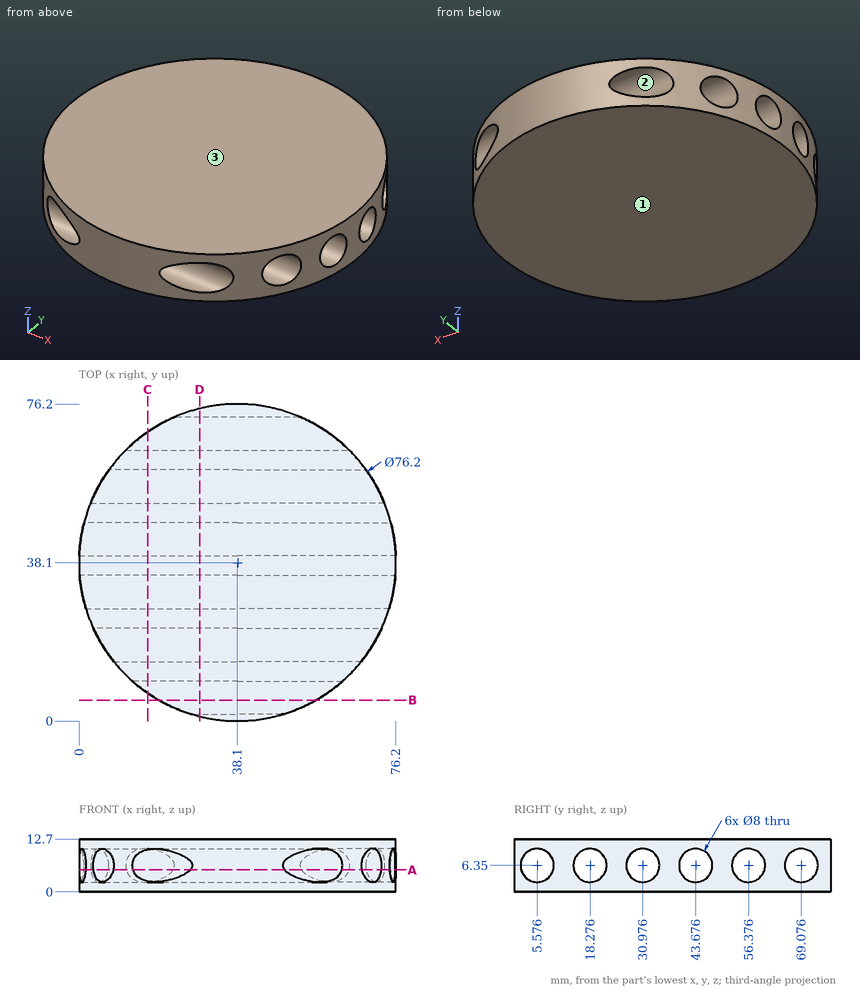
The drawing under review shows one solid part. Ordinate dimensions are in mm from its lowest x, y, z. Round coordinates to 2 decimals unless told otherwise and drop trailing zeros. Write each loop counter-clockwise with the first axis right and the second up, starting at its lowest first coordinate (ties: lowest second). Pieces come first, ordered by that corner, then holes. Notation, with made-up numbers: (15, 35.25) - (36, 35.25) arc R11 ccw to (36, 52.25) - close; hole circle Ø6 at (-37.5, 34). An arc over 180 degrees is marked (long way). One line per question, with ' | ' between items.
Item 1: The part is to be moulded in two halves that separate along Z. For the marked faces 1, 2 and 3, say which applies: pulls with the +Z half, pulls with the -Z half, needs draft (parallel to the pull), parting line crosses it, or undercut.
Resolved:
face 1: pulls with the -Z half | face 2: undercut | face 3: pulls with the +Z half
Item 2: Add section B-B, the plane y = 5. Give the boundary of the cut face in (x, z), then the cut area to 4 significant figures.
Resolved:
outline: (19.23, 0) - (56.97, 0) - (56.97, 2.39) - (19.23, 2.39) - close; (19.23, 10.31) - (56.97, 10.31) - (56.97, 12.7) - (19.23, 12.7) - close | area: 180.5 mm2
Item 3: To check wall thickness, follow probe 1 along Y at (x, z) = (72, 5); probe 2 along Y at (x, z) = (10.5, 5.25) (1 decimal); probe 3 along Y at (x, z) = (57, 7.75). State the ranges of each line that lie inside material, in increasing order.
Resolved:
probe 1: y = 22.04 to 27.21, 34.74 to 39.91, 47.44 to 52.61 | probe 2: y = 11.8 to 14.4, 22.1 to 27.1, 34.8 to 39.8, 47.5 to 52.5, 60.2 to 64.4 | probe 3: y = 9.32 to 14.53, 22.02 to 27.23, 34.72 to 39.93, 47.42 to 52.63, 60.12 to 65.33
Item 4: Add section A-A, the plane z = 5.25. Give the boundary of the cut face in (x, y).
Resolved:
outline: (0.04, 39.83) arc R38.1 ccw to (0.14, 34.82) - (76.06, 34.82) arc R38.1 ccw to (76.16, 39.83) - close; (1.18, 47.52) - (75.02, 47.52) arc R38.1 ccw to (73.36, 52.53) - (2.84, 52.53) arc R38.1 ccw to start; (1.61, 27.13) arc R38.1 ccw to (3.51, 22.12) - (72.69, 22.12) arc R38.1 ccw to (74.59, 27.13) - close; (7.08, 60.22) - (69.12, 60.22) arc R38.1 ccw to (64.85, 65.23) - (11.35, 65.23) arc R38.1 ccw to start; (8.24, 14.43) arc R38.1 ccw to (13.02, 9.42) - (63.18, 9.42) arc R38.1 ccw to (67.96, 14.43) - close; (22.64, 72.92) - (53.56, 72.92) arc R38.1 ccw to start; (26.75, 1.73) arc R38.1 ccw to (49.45, 1.73) - close
Item 5: Add section C-C, the plane x = 16.5. Give the boundary of the cut face in (y, z), then the cut area to 3 significant figures.
Resolved:
outline: (6.71, 0) - (69.49, 0) - (69.49, 2.37) arc R4 cw (long way) to (69.49, 10.33) - (69.49, 12.7) - (6.71, 12.7) - (6.71, 10.18) arc R4 cw to (6.71, 2.52) - close; hole circle Ø8 at (18.28, 6.35); hole circle Ø8 at (30.98, 6.35); hole circle Ø8 at (43.68, 6.35); hole circle Ø8 at (56.38, 6.35) | area: 552 mm2
Item 6: For P1, Ø6, axis at x = 63, y = 9, coming from the +Z side; P2, Ø5, axis at y = 69.08, z = 6.35, coming from the +X side; P3, Ø3, axis at y = 23, z = 1.5, coming from the -X side; P4, Ø3, axis at x = 64, z = 7.5, coming from the +Y side, all flat-tipped, find the tip position at first contact; note any pin that passes through.
Resolved:
P1: stops at z = 12.7 | P2: passes through | P3: stops at x = 2.51 | P4: stops at y = 66.08
Item 7: Add section D-D, the plane x = 29. Give the boundary of the cut face in (y, z).
Resolved:
outline: (1.1, 0) - (75.1, 0) - (75.1, 12.7) - (1.1, 12.7) - close; hole circle Ø8 at (5.58, 6.35); hole circle Ø8 at (18.28, 6.35); hole circle Ø8 at (30.98, 6.35); hole circle Ø8 at (43.68, 6.35); hole circle Ø8 at (56.38, 6.35); hole circle Ø8 at (69.08, 6.35)
